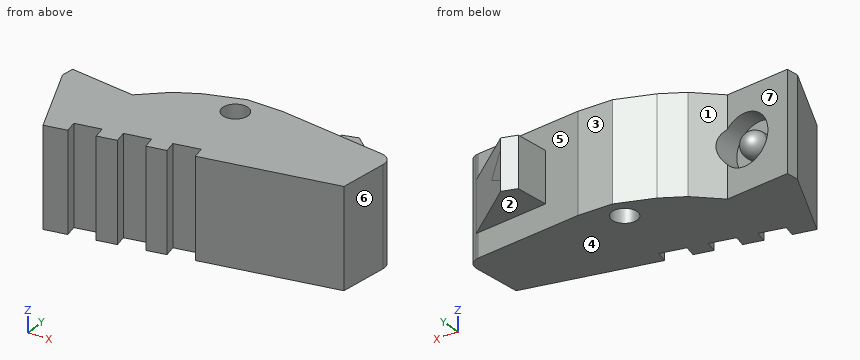
```python
from build123d import *

# Parameters (mm, degrees)
SKETCH_2_R          = 1
EXTRUDE_2_DEPTH     = 7.8
SKETCH_3_W          = 6
SKETCH_3_H          = 4
EXTRUDE_3_DEPTH     = 4
CHAMFER_1_SIZE      = 1.3
CHAMFER_1_SIZE2     = 3
CHAMFER_2_SIZE      = 6.159459855
CHAMFER_2_SIZE_2    = 4
SKETCH_4_R          = 2
CUT_EXTRUDE_1_DEPTH = 1.5
SKETCH_5_R          = 1
EXTRUDE_4_DEPTH     = 1.5
FILLET_1_R          = 1
SKETCH_6_W          = 2
SKETCH_6_H          = 7.8
CUT_EXTRUDE_2_DEPTH = 1
FILLET_START        = -1
FILLET_2_DEPTH      = 10
FILLET_2_2_DEPTH    = 2.9
FILLET_START_2      = 5.9
FILLET_2_3_DEPTH    = 3.1


with BuildPart() as part:
    # 스케치2 → 보스-돌출2 (new body)
    with BuildSketch(Plane.XY):
        Polygon((2.5, 1.75), (12.045629808, 0.577944035), (11.448632524, -4.284208661), (-9.375446541, -8.532579884), (-12.070254037, -2.279394966), (-11.94829225, -1.286095926), (-6.802600831, -1.917907388), (-4.857687993, -0.185790939), (-3.065051347, 0.78210453), (-0.230903775, 1.75), align=None)
        Circle(SKETCH_2_R, mode=Mode.SUBTRACT)
    extrude(amount=EXTRUDE_2_DEPTH)

    # 스케치3 → 보스-돌출3 (add)
    with BuildSketch(Plane(origin=(0.248812001, 2.02641113, 0), x_dir=(0.9925461516413224, -0.12186934340514406, 0), z_dir=(0.12186934340514406, 0.9925461516413224, 0))):
        with Locations((8.062111671, -3.9)):
            Rectangle(SKETCH_3_W, SKETCH_3_H)
    extrude(amount=EXTRUDE_3_DEPTH)

    # 모따기1
    chamfer_1_edges = [part.edges().sort_by_distance(p)[0] for p in [
        (5.760668833, 5.379679511, 3.9),
    ]]
    chamfer_1_side = [part.faces().sort_by_distance(p)[0] for p in [
        (5.516930146, 3.394587208, 3.9),
    ]]
    chamfer(chamfer_1_edges, length=CHAMFER_1_SIZE, length2=CHAMFER_1_SIZE2, reference=chamfer_1_side[0])

    # 모따기2
    # the kernel refuses this chamfer: 6.159459855, 4 mm, written as the material it takes off along each edge
    with BuildSketch(Plane(origin=(9.288459468, -15.121825718, 5.9), x_dir=(-0.9925461516413224, 0.12186934340514405, 0), z_dir=(0.12186934340514406, 0.9925461516413224, 0))) as chamfer_2_piece_1_section:
        Polygon((CHAMFER_2_SIZE, 0), (0, -CHAMFER_2_SIZE_2), (0, 0), align=None)
    chamfer_2_piece_1 = extrude(amount=35.837521179, mode=Mode.PRIVATE)
    chamfer_2_piece_1 = split(chamfer_2_piece_1, bisect_by=Plane(origin=(17.870057149, -4.894675852, 5.9), z_dir=(0.6427876096865351, 0.7660444431189816, 0)), keep=Keep.TOP, mode=Mode.PRIVATE)
    add(chamfer_2_piece_1, mode=Mode.SUBTRACT)
    with BuildSketch(Plane(origin=(9.288459468, -15.121825718, 1.9), x_dir=(-0.9925461516413225, 0.12186934340514408, 0), z_dir=(0.12186934340514406, 0.9925461516413224, 0))) as chamfer_2_piece_2_section:
        Polygon((CHAMFER_2_SIZE, 0), (0, CHAMFER_2_SIZE_2), (0, 0), align=None)
    chamfer_2_piece_2 = extrude(amount=35.837521179, mode=Mode.PRIVATE)
    chamfer_2_piece_2 = split(chamfer_2_piece_2, bisect_by=Plane(origin=(17.870057149, -4.894675852, 1.9), z_dir=(0.6427876096865351, 0.7660444431189816, 0)), keep=Keep.TOP, mode=Mode.PRIVATE)
    add(chamfer_2_piece_2, mode=Mode.SUBTRACT)
    with BuildSketch(Plane(origin=(11.715945743, 4.648463451, -14.01876059), x_dir=(-0.9925461516413225, 0.1218693434051441, 0), z_dir=(0, 0, 1))) as chamfer_2_piece_3:
        Polygon((CHAMFER_2_SIZE, 0), (0, CHAMFER_2_SIZE_2), (0, 0), align=None)
    extrude(amount=35.837521179, mode=Mode.SUBTRACT)

    # 스케치4 → 컷-돌출1 (cut, symmetric)
    with BuildSketch(Plane(origin=(-0.333025054, -2.712271409, 0), x_dir=(0.9925461516413224, -0.12186934340514398, 0), z_dir=(0.12186934340514398, 0.9925461516413224, 0))):
        with Locations(Location((-8.018161162, -3.9, 0), (0, 0, 180))):
            Circle(SKETCH_4_R)
    extrude(amount=CUT_EXTRUDE_1_DEPTH, both=True, mode=Mode.SUBTRACT)

    # 스케치5 → 보스-돌출4 (add)
    with BuildSketch(Plane(origin=(-0.515829069, -4.201090636, 0), x_dir=(0.9925461516413224, -0.12186934340514398, 0), z_dir=(0.12186934340514398, 0.9925461516413224, 0))):
        with Locations(Location((-8.018161162, -3.9, 0), (0, 0, 180))):
            Circle(SKETCH_5_R)
    extrude(amount=EXTRUDE_4_DEPTH)

    # 필렛1
    fillet_1_edges = [part.edges().sort_by_distance(p)[0] for p in [
        (-7.298873907, -1.856972716, 3.9),
    ]]
    fillet(fillet_1_edges, radius=FILLET_1_R)

    # 스케치6 → 컷-돌출2 (cut)
    with BuildSketch(Plane(origin=(1.296571576, -6.355355406, 0), x_dir=(0.9798173389697206, 0.19989492803544545, 0), z_dir=(0.19989492803544545, -0.9798173389697206, 0))):
        with Locations((-8.133925678, 3.9)):
            Rectangle(SKETCH_6_W, SKETCH_6_H)
        with Locations((-4.633925678, 3.9)):
            Rectangle(SKETCH_6_W, SKETCH_6_H)
        with Locations((-1.133925678, 3.9)):
            Rectangle(SKETCH_6_W, SKETCH_6_H)
    extrude(amount=-CUT_EXTRUDE_2_DEPTH, mode=Mode.SUBTRACT)

    # 필렛2: read off the stored shape, not the designer's step
    # 필렛2 outline → 필렛2 (cut)
    with BuildSketch(Plane.XY.offset(FILLET_START)):
        with BuildLine():
            Line((11.228468369, 0.678278844), (11.260303349, 0.651566124))
            ThreePointArc((11.260303349, 0.651566124), (11.780248218, 0.235605593), (11.923760465, -0.414602116))
            Line((11.923760465, -0.414602116), (12.045629808, 0.577944035))
            Line((12.045629808, 0.577944035), (11.228468369, 0.678278844))
        make_face()
    extrude(amount=FILLET_2_DEPTH, mode=Mode.SUBTRACT)

    # Fillet 2 2 outline → Fillet 2 2 (cut)
    with BuildSketch(Plane.XY.offset(FILLET_START)):
        with BuildLine():
            Line((11.228468369, 0.678278844), (11.053083657, 0.699813379))
            ThreePointArc((11.053083657, 0.699813379), (11.157980304, 0.6812165), (11.260303349, 0.651566124))
            Line((11.260303349, 0.651566124), (11.228468369, 0.678278844))
        make_face()
    extrude(amount=FILLET_2_2_DEPTH, mode=Mode.SUBTRACT)

    # Fillet 2 3 outline → Fillet 2 3 (cut)
    with BuildSketch(Plane.XY.offset(FILLET_START_2)):
        with BuildLine():
            Line((11.228468369, 0.678278844), (11.053083657, 0.699813379))
            ThreePointArc((11.053083657, 0.699813379), (11.157980304, 0.6812165), (11.260303349, 0.651566124))
            Line((11.260303349, 0.651566124), (11.228468369, 0.678278844))
        make_face()
    extrude(amount=FILLET_2_3_DEPTH, mode=Mode.SUBTRACT)


solid = part.part
```
The model under review builds one solid part; all positions refer to its coordinate system, in mm. Face numbers are marked on the shaded views. A direction names the side the tool comes from. Give positions to 0.01 mm unless a question says otherwise; leave off trailing zeros. Write each loop counter-clockwise with the first axis right and the second up, starting at its lowest first coordinate (ties: lowest second). Pieces come first, ordered by that corner, then holes. Notation, with made-up numbers: (47.5, 24) - (58.5, 24) arc R26 cw to (58.5, 43) - close; hole circle Ø1 at (45, -40). An arc over 180 degrees is marked (long way). Answer in a Markdown table with one row per item. Add a question column.
1. We need section B-B on x = 0. Write out the cut boundary in (y, z), then the cut area to 3 significant figures.
2. Wall thickness on line 1 along Y through (x, z) = (0, 2.75); line 2 along Y through (x, z) = (-9, 5.25); line 3 along Y through (x, z) = (-5.25, 7.75): over which ranges is each line inside the solid? List them lowest first. Write a range as [from, to].
3. Tool access review of the marked faces 1, 2 and 3: name each direction out of +Z, -Z, +X, -X, +Y, -Y from which nothing blocks a thin tool from reaching the whole face with its end or side.
4. Insertion check: P1, Ø2, axis at x = 1.5, z = 2.5, coming from the +Y side; P2, Ø1, axis at x = -4.5, z = 5.5, coming from the -Y side; P3, Ø1.9, axis at x = 8.5, y = 2.5, coming from the -Z side. Each pin has a flat end and moves straight along its axis. Give the tip position at first contact, or say it passes through.
5. We need section D-D on x = 2.75. Write out the cut boundary in (y, z).
6. We need section A-A on z = 0.75. Write out the cut boundary in (x, y).
7. Draft analysis for pull direction X (two halves, no side actions). For the marked faces 4, 5, 6 and 7, state which applies: +X half, -X half, draft (parallel to the pull), parting line (faces both ways), or undercut.
Ans:
| question | item | result |
|---|---|---|
| 1 | outline | (-5.6, 0) - (-1, 0) - (-1, 7.8) - (-5.6, 7.8) - close; (1, 0) - (1.75, 0) - (1.75, 7.8) - (1, 7.8) - close |
| 1 | area | 41.7 mm^2 |
| 2 | line 1 | y = [-5.6, -1], [1, 1.75] |
| 2 | line 2 | y = [-8.46, -3.16] |
| 2 | line 3 | y = [-7.69, -0.54] |
| 3 | face 1 | +Z, -Z, +Y |
| 3 | face 2 | -Z, +X, +Y |
| 3 | face 3 | +Z, -Z, -X, +Y |
| 4 | P1 | stops at y = 1.75 |
| 4 | P2 | stops at y = -7.64 |
| 4 | P3 | stops at z = 1.9 |
| 5 | outline | (-6.06, 0) - (1.72, 0) - (1.72, 7.8) - (-6.06, 7.8) - close |
| 6 | outline | (-12.07, -2.28) - (-9.38, -8.53) - (-7.65, -8.18) - (-7.85, -7.2) - (-5.89, -6.8) - (-5.69, -7.78) - (-4.22, -7.48) - (-4.42, -6.5) - (-2.46, -6.1) - (-2.26, -7.08) - (-0.79, -6.78) - (-0.99, -5.8) - (0.97, -5.4) - (1.17, -6.38) - (11.45, -4.28) - (11.92, -0.41) arc R1 ccw to (11.05, 0.7) - (2.5, 1.75) - (-0.23, 1.75) - (-3.07, 0.78) - (-4.86, -0.19) - (-6.8, -1.92) - (-11.95, -1.29) - close; hole circle Ø2 at (0, 0) |
| 7 | face 4 | draft |
| 7 | face 5 | undercut |
| 7 | face 6 | +X half |
| 7 | face 7 | undercut |
